Input: part model. Units: mm. Frame: model coordinates. Face numbers are marked on the shaded views. Coordinates: 2 decimals unless noted, no trailing zeros. Loops run counter-clockwise (first coordinate to the right, second up) from the corner with the lowest first, then second, coordinate; pieces in that order, holes last.
(1) Line query: L1, parallel to X at y = 0, z = 8.5 (3 decimals); L2, parallel to Y at x = -35, z = 10.25 (3 decimals); L3, parallel to Z at x = -5.5, y = -1. Output: solid intervals per line, ascending.
(2) Section C-C, the plane y = 0. Return loops of the section in (x, z) (3 decimals), then the cut area to 3 significant figures.
(3) Section A-A, the plane z = 8.75. Return loops of the section in (x, y) (3 decimals).
(4) Mould query, pull axis X, two halves, no side actions, for the marked faces 1 and 2. Classes: released by +X, released by -X, zero draft, split by the parting line, or undercut.
(5) Section B-B, the plane x = 35. Return loops of the section in (y, z) (3 decimals).
(6) Contact query for flat-ended pins moving along their axis: P1, Ø5, axis at x = -40, y = 12, coming from the +Z side; P2, Ø5, axis at y = 3.5, z = 10.5, coming from the -X side. Output: stop coordinate, or through.
(7) Section D-D, the plane y = 5. Return loops of the section in (x, z).
Autodesk Inventor part; units mm, degrees
ref_plane "YZ Plane" through (0, 0, 0) normal (1, 0, 0) x (0, 1, 0)
ref_plane "XZ Plane" through (0, 0, 0) normal (0, 1, 0) x (-1, 0, 0)
ref_plane "XY Plane" through (0, 0, 0) normal (0, 0, 1) x (1, 0, 0)
sketch "Náčrt1" plane through (0, 0, 0) normal (0, 0, 1) x (1, 0, 0)
  line L0 (0, 21) -> (0, -21)
  line L1 (-70, 0) -> (70, 0)
  line L2 (-50, 15) -> (50, 15)
  line L3 (50, 15) -> (50, -15)
  line L4 (50, -15) -> (-50, -15)
  line L5 (-50, -15) -> (-50, 15)
  point P0 (0, 0)
  dimension "d0" = 100
  dimension "d1" = 30
extrude "Vysunutí1" add sketch "Náčrt1" along normal blind 2.5
sketch "Náčrt2" plane through (0, 0, 2.5) normal (0, 0, 1) x (1, 0, 0)
  line L0 (-50, -15) -> (50, -15)
  line L1 (50, -15) -> (50, 15)
  line L2 (50, 15) -> (-50, 15)
  line L3 (-50, 15) -> (-50, -15)
  line L4 (0, 21) -> (0, -21)
  line L5 (-70, 0) -> (70, 0)
  circle A0 centre (35, 0) radius 1.5
  circle A1 centre (35, 0) radius 2.575
  circle A2 centre (-35, 0) radius 1.5
  circle A3 centre (-35, 0) radius 2.575
  point P0 (0, 0)
  point P1 (50, 0)
  dimension "d11" = 3
  dimension "d12" = 5.15
  dimension "d13" = 15
fillet "Zaoblení1" radius 2 4 edges at (50, 0, 0) (0, 15, 0) (-50, 0, 0) (0, -15, 0)
fillet "Zaoblení2" radius 1 8 edges at (50, -15, 2.25) (49.4142, -14.4142, 0.5858) (50, 15, 2.25) (49.4142, 14.4142, 0.5858) (-50, 15, 2.25) (-49.4142, 14.4142, 0.5858) (-50, -15, 2.25) (-49.4142, -14.4142, 0.5858)
extrude "Vysunutí3" add sketch "Náčrt2" along normal blind 10 contours A3 L5 A2 | L5 A2 A3 | A1 L5 A0 | L5 A0 A1
properties part number "záslepka_3D tisk"
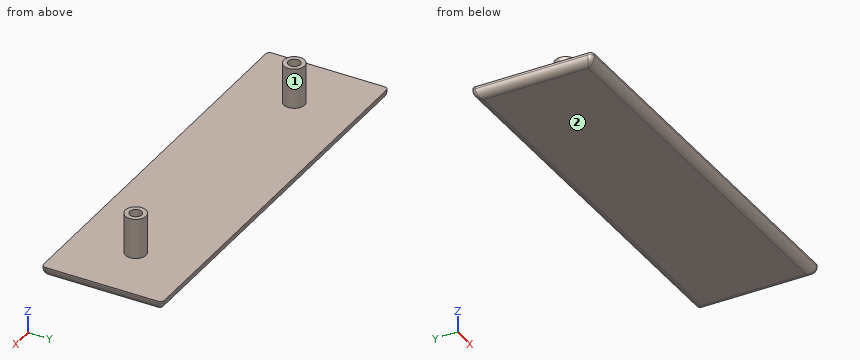
Report:
1. L1: x = -37.575 to -36.5, -33.5 to -32.425, 32.425 to 33.5, 36.5 to 37.575
1. L2: y = -2.575 to -1.5, 1.5 to 2.575
1. L3: z = 0 to 2.5
2. outline: (-50, 2) arc R2 ccw to (-48, 0) - (48, 0) arc R2 ccw to (50, 2) - (50, 2.5) - (37.575, 2.5) - (37.575, 12.5) - (36.5, 12.5) - (36.5, 2.5) - (33.5, 2.5) - (33.5, 12.5) - (32.425, 12.5) - (32.425, 2.5) - (-32.425, 2.5) - (-32.425, 12.5) - (-33.5, 12.5) - (-33.5, 2.5) - (-36.5, 2.5) - (-36.5, 12.5) - (-37.575, 12.5) - (-37.575, 2.5) - (-50, 2.5) - close
2. area: 291 mm2
3. outline: circle Ø5.15 at (-35, 0); circle Ø5.15 at (35, 0); hole circle Ø3 at (-35, 0); hole circle Ø3 at (35, 0)
4. face 1: undercut
4. face 2: zero draft
5. outline: (-15, 2) arc R2 ccw to (-13, 0) - (13, 0) arc R2 ccw to (15, 2) - (15, 2.5) - (2.575, 2.5) - (2.575, 12.5) - (1.5, 12.5) - (1.5, 2.5) - (-1.5, 2.5) - (-1.5, 12.5) - (-2.575, 12.5) - (-2.575, 2.5) - (-15, 2.5) - close
6. P1: stops at z = 2.5
6. P2: stops at x = -37.37
7. outline: (-50, 2) arc R2 ccw to (-48, 0) - (48, 0) arc R2 ccw to (50, 2) - (50, 2.5) - (-50, 2.5) - close
